Part print with two shaded views. Sizes in mm from the minimum x, y, z corner. A direction names the side the tool comes from. Round coordinates to 2 decimals unless told otherwise and drop trailing zeros. Order: outer loops, then holes, each group sorted by start corner. A loop starts at its lowest first (then second) coordinate and runs counter-clockwise, first axis right, second up. Notation, with made-up numbers: M 25.25,73.25 L 34.25,73.25 A16 cw 34.25,92.25 Z; hole C 68,50.25 d2. An arc over 180 degrees is marked long. Answer as a JSON object with one key per item and string values.
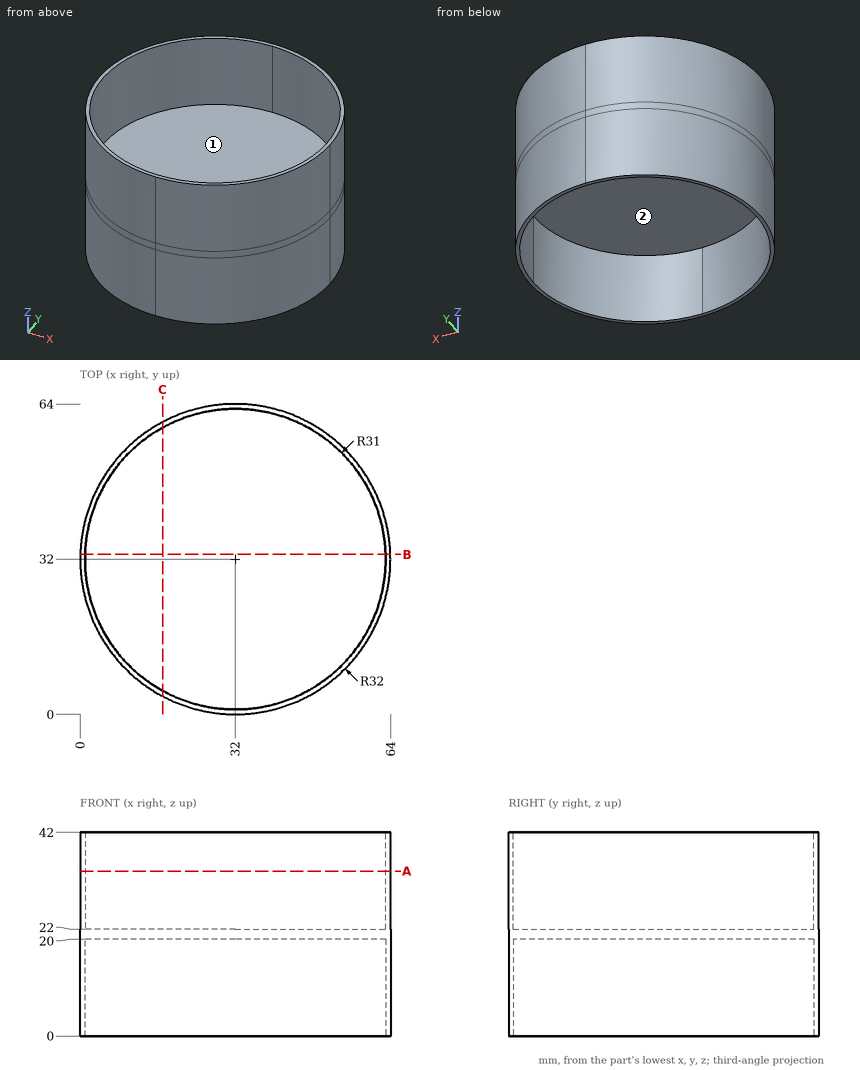
Item 1: Saw through at B-B on y = 33. List the corners of the cut face in (x, z).
Worked answers:
{"outline": "M 0.02,0 L 1.02,0 L 1.02,20 L 62.98,20 L 62.98,0 L 63.98,0 L 63.98,42 L 62.98,42 L 62.98,22 L 1.02,22 L 1.02,42 L 0.02,42 Z"}
Item 2: Saw through at C-C on x = 17. List the corners of the cut face in (y, z).
Worked answers:
{"outline": "M 3.73,0 L 4.87,0 L 4.87,20 L 59.13,20 L 59.13,0 L 60.27,0 L 60.27,42 L 59.13,42 L 59.13,22 L 4.87,22 L 4.87,42 L 3.73,42 Z"}
Item 3: Wall check: line 1 along X through (y, z) = (32, 30); line 2 along Z through (x, y) = (18.5, 57.5); line 3 along Y through (x, z) = (4, 6.5). Give the ranges that are in metal, low to high. Write a range as [from, to].
Worked answers:
{"line 1": "x = [0, 1], [63, 64]", "line 2": "z = [20, 22]", "line 3": "y = [16.51, 18.7], [45.3, 47.49]"}
Item 4: Drop flat-ended pins along their axis: pin 1 Ø6 at (x, y) = (25, 15.5) entering from +Z; pin 2 Ø1.5 at (x, z) = (48.5, 8.5) entering from +Y; pin 3 Ø12 at (y, z) = (33, 27.5) entering from -X. Give the stop position or say it passes through.
Worked answers:
{"pin 1": "stops at z = 22", "pin 2": "stops at y = 59.86", "pin 3": "stops at x = 0"}
Item 5: 3-axis set-ups, long thin cutter, end or side, ignore diameter. For the marked faces 1 and 2: which of +Z, -Z, +X, -X, +Y, -Y reach the whole face in a straight line?
Worked answers:
{"face 1": "+Z", "face 2": "-Z"}
Item 6: Saw through at A-A on z = 34. List the corners of the cut face in (x, y), and give its area (3 significant figures).
Worked answers:
{"outline": "C 32,32 d64; hole M 32,63 A31 ccw long 63,32 A31 ccw Z", "area": "198 mm2"}
